```python
from build123d import *

# Parameters (mm, degrees)
SKETCH2_W         = 19.3548
SKETCH2_H         = 2.3876
SLOT_DEPTH        = 2.2352
CIRPATTERN1_COUNT = 2
CIRPATTERN1_ANGLE = 90


with BuildPart() as part:
    # BodySke → Base-Revolve (revolve)
    with BuildSketch(Plane.XY, mode=Mode.PRIVATE) as base_revolve_sk:
        Polygon((0, 0), (0, 9.6774), (0.188054315, 9.6774), (5.842, 4.7625), (38.1, 4.7625), (38.1, 0), align=None)
    revolve(base_revolve_sk.sketch.rotate(Axis((-6.35, 0, 0), (1, 0, 0)), 90), axis=Axis((-6.35, 0, 0), (1, 0, 0)))

    # Sketch2 → Slot (cut)
    with BuildSketch(Plane.ZY):
        Rectangle(SKETCH2_W, SKETCH2_H)
    extrude(amount=-SLOT_DEPTH, mode=Mode.SUBTRACT)

    # Sketch3 → Cross section 0
    with BuildSketch(Plane.ZY):
        with BuildLine():
            Line((-1.0922, 6.6421), (1.0922, 6.6421))
            Line((1.0922, 6.6421), (1.0922, -6.6421))
            Line((1.0922, -6.6421), (-1.0922, -6.6421))
            Line((-1.0922, -6.6421), (-1.0922, 6.6421))
        make_face()
    # Sketch4 → Cross section 1
    with BuildSketch(Plane.ZY.offset(-7.9756)):
        with BuildLine():
            Line((-0.5461, 0.5461), (0.5461, 0.5461))
            Line((0.5461, 0.5461), (0.5461, -0.5461))
            Line((0.5461, -0.5461), (-0.5461, -0.5461))
            Line((-0.5461, -0.5461), (-0.5461, 0.5461))
        make_face()
    cross = loft(mode=Mode.SUBTRACT)

    # CirPattern1: Cross ×2 about axis
    cirpattern1_axis = Axis((0, 0, 0), (1, 0, 0))
    for i in range(1, CIRPATTERN1_COUNT):
        add(cross.rotate(cirpattern1_axis, i * CIRPATTERN1_ANGLE / (CIRPATTERN1_COUNT - 1)), mode=Mode.SUBTRACT)


solid = part.part
```
CAD build for the part. Positions are in the model's coordinates, mm. A direction names the side the tool comes from. Give positions to 0.01 mm unless a question says otherwise; leave off trailing zeros. Write each loop counter-clockwise with the first axis right and the second up, starting at its lowest first coordinate (ties: lowest second). Pieces come first, ordered by that corner, then holes. Notation, with made-up numbers: M -2,57.25 L 20,57.25 A13 cw 20,76.25 Z; hole C -19,79 d9. An arc over 180 degrees is marked long. Return JSON: item names as keys, results as strings. Group by question number.
(1) Drill centre lines: L1, parallel to Y at x = 4, z = -1; L2, parallel to Y at x = 26, z = 0; L3, parallel to Y at x = 6.5, z = 0.5. Where is each one in solid material? Low to high. Write a range as [from, to].
(2) Flat gauge pins, fed straight in: pin 1 Ø5 at (y, z) = (0, -3.5) entering from -X; pin 2 Ø8 at (x, z) = (27.5, -2) entering from +Y; pin 3 Ø0.9 at (y, z) = (0, 0) entering from -X; pin 4 Ø1 at (x, z) = (12, 4.5) entering from -Y. Where does each tip first touch, or does it go through?
(3) Band-saw the part on A-A (x = 16). Give the cut face in (y, z) (1 decimal).
(4) Mould opens along Y. For faces 1 (the face through (1, 1.194, 5)), 2 (the face through (0, 4, -2)), 3 (the face through (5.57, -1.5, 4.77)) say: pulls with the +Y half, pulls with the -Y half, needs draft (parallel to the pull), parting line crosses it, or undercut.
(5) 3-axis set-ups, long thin cutter, end or side, ignore diameter. For faces 4 (the face through (7.976, 0, 0)), 5 (the face through (38.1, 0, 0)), 6 (the face through (1, 1.194, -5)), 7 (the face through (22.2, 4.65, -1.03)): which of +Z, -Z, +X, -X, +Y, -Y reach the whole face in a straight line?
Entries:
{
 "1": {"L1": "y = [-6.28, -0.82], [0.82, 6.28]", "L2": "y = [-4.76, 4.76]", "L3": "y = [-4.74, -1.67], [1.67, 4.74]"},
 "2": {"pin 1": "stops at x = 0", "pin 2": "stops at y = 4.76", "pin 3": "stops at x = 7.98", "pin 4": "stops at y = -2.58"},
 "3": {"outline": "C 0,0 d9.5"},
 "4": {"face 1": "undercut", "face 2": "needs draft", "face 3": "parting line crosses it"},
 "5": {"face 4": "-X", "face 5": "+Z, -Z, +X, +Y, -Y", "face 6": "+Z, -Z, -X", "face 7": "+X"}
}
